For this review, take the finished solid that the model builds, in its own axes (mm). A direction names the side the tool comes from. Round coordinates to 2 decimals unless told otherwise and drop trailing zeros. Use one line per item in the form item = value. Start each with the question number.
Item 1: For line 1 (X direction, y = 30.5, z = -1.25); line 2 (Y direction, x = 24.5, z = -2); line 3 (Y direction, x = 47, z = 0.5), list the stretches that pass through material, from the lowest coordinate up. Write a range as [from, to].
Item 2: For faces 5 (the flat face through (-1, 1, -12.7)), 6 (the flat face through (-36.32, -4.3, 5.82)), list the 3-axis set-ups (+Z, -Z, +X, -X, +Y, -Y) from which the entire face can be reached by the end or side of a thin tool; tool diameter is ignored.
Item 3: Draft analysis for pull direction X (two halves, no side actions). For faces 1 (the flat face through (-28.723, 22.639, 5.822)), 2 (the cylindrical face through (-48.29, -11.48, -2.48)), 3 (the flat face through (-56.031, 23.084, -0.116)), 4 (the flat face through (56.031, -23.084, -0.116)), state which applies: released by +X, released by -X, zero draft, split by the parting line, or undercut.
Item 4: For P1, Ø5, axis at y = 38, z = -7, coming from the +X side; P2, Ø12, axis at x = 12, z = 7.5, coming from the -Y side; P3, Ø4, axis at y = -3, z = -6, coming from the -X side, all flat-tipped, find the tip position at first contact; note any pin that passes through.
from build123d import *

# Parameters (mm, degrees)
SKETCH1_R           = 38.1
BOSS_EXTRUDE1_DEPTH = 12.7
SKETCH2_OUTSIDE_W   = 100.344
SKETCH2_OUTSIDE_H   = 100.344
CUT_EXTRUDE1_DEPTH  = 25.4
SKETCH3_R           = 8.255
BOSS_EXTRUDE2_DEPTH = 25.4
CIRPATTERN4_COUNT   = 8
CHAMFER2_SIZE       = 2.54


with BuildPart() as part:
    # Sketch1 → Boss-Extrude1 (new body, symmetric)
    with BuildSketch(Plane.XY):
        Circle(SKETCH1_R)
    extrude(amount=BOSS_EXTRUDE1_DEPTH, both=True)

    # Sketch2 outside → Cut-Extrude1 (cut)
    with BuildSketch(Plane.XY.offset(12.7)):
        Rectangle(SKETCH2_OUTSIDE_W, SKETCH2_OUTSIDE_H)
        Polygon((38.1, 0), (26.940768363, 26.940768363), (0, 38.1), (-26.940768363, 26.940768363), (-38.1, 0), (-26.940768363, -26.940768363), (0, -38.1), (26.940768363, -26.940768363), align=None, mode=Mode.SUBTRACT)
    extrude(amount=-CUT_EXTRUDE1_DEPTH, mode=Mode.SUBTRACT)

    # Sketch3 → Boss-Extrude2 (add)
    with BuildSketch(Plane(origin=(13.470384182, 32.520384182, 0), x_dir=(0.923879533, -0.382683432, 0), z_dir=(0.382683432, 0.923879533, 0))):
        Circle(SKETCH3_R)
    boss_extrude2 = extrude(amount=BOSS_EXTRUDE2_DEPTH)

    # CirPattern4: Boss-Extrude2 ×8 about axis
    cirpattern4_axis = Axis((0, 0, 0), (0, 0, 1))
    for i in range(1, CIRPATTERN4_COUNT):
        add(boss_extrude2.rotate(cirpattern4_axis, i * 360 / CIRPATTERN4_COUNT))

    # Chamfer2
    chamfer2_edges = [part.edges().sort_by_distance(p)[0] for p in [
        (5.843758641, 35.679435916, 0),
        (29.361332447, 21.097009722, 0),
        (35.679435916, -5.843758641, 0),
        (21.097009722, -29.361332447, 0),
        (-5.843758641, -35.679435916, 0),
        (-29.361332447, -21.097009722, 0),
        (-35.679435916, 5.843758641, 0),
        (-21.097009722, 29.361332447, 0),
    ]]
    chamfer(chamfer2_edges, length=CHAMFER2_SIZE)


solid = part.part
Calculated:
q1.line_1 = [-52.96, -52.31], [-22.5, 22.5], [52.31, 52.96]
q1.line_2 = [-55.44, -38.22], [-27.95, 27.95], [38.22, 55.44]
q1.line_3 = [-28.39, -10.55], [10.55, 28.39]
q2.face_5 = -Z, +X, -X, +Y, -Y
q2.face_6 = none
q3.face_1 = undercut
q3.face_2 = undercut
q3.face_3 = released by -X
q3.face_4 = released by +X
q4.P1 = 23.5
q4.P2 = -58.9
q4.P3 = -37.69
